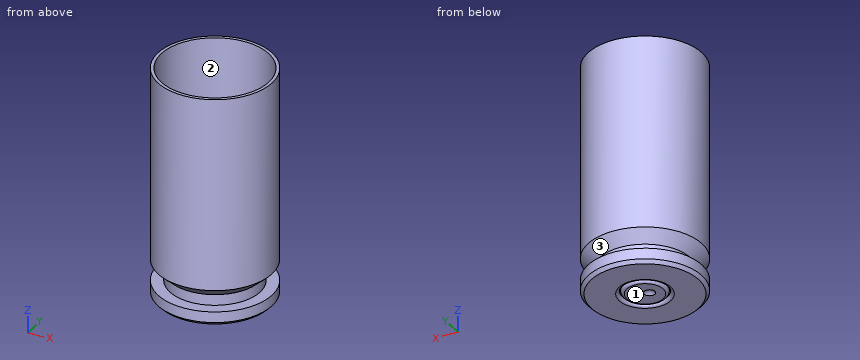
from build123d import *

# Parameters (mm, degrees)
F2_R    = 2
F3_R    = 0.3
F4_SIZE = 0.3


with BuildPart() as f1:
    # F0 (on Front) → F1 (revolve)
    with BuildSketch(Plane.XZ):
        Polygon((2.1, 0), (5.3, 0), (5.3, 1.3), (4.2, 1.3), (4.2, 2.3), (5.3, 3.3), (5.3, 21.25), (5, 21.25), (5, 3.378872), (0.63314, 3.378872), (0.63314, 1.22387), (0, 1.22387), (0, 0), (2, 0), (2, 0.961065), (2.1, 0.961065), align=None)
    revolve(axis=Axis((0, 0, 10.625), (0, 0, 1)))

    # F2
    f2_edges = [f1.edges().sort_by_distance(p)[0] for p in [
        (-5, 0, 3.378872),
    ]]
    fillet(f2_edges, radius=F2_R)

    # F3
    f3_edges = [f1.edges().sort_by_distance(p)[0] for p in [
        (-2.1, 0, 0),
        (-2, 0, 0),
    ]]
    fillet(f3_edges, radius=F3_R)

    # F4
    f4_edges = [f1.edges().sort_by_distance(p)[0] for p in [
        (-5.3, 0, 0),
    ]]
    chamfer(f4_edges, length=F4_SIZE)

    # F5 (on Front) → F6 (revolve, cut)
    with BuildSketch(Plane.XZ):
        with BuildLine():
            Line((-0.916817, 0), (-0.416817, 0))
            Line((-0.416817, 0), (-0.416817, 0.205113))
            ThreePointArc((-0.416817, 0.205113), (-0.687035, 0.151842), (-0.916817, 0))
        make_face()
    revolve(axis=Axis((-0.416817, 0, 0.102557), (0, 0, 1)), mode=Mode.SUBTRACT)


solid = f1.part
Design review of the part built by this model. Coordinates are the model's own, in mm. Face numbers are marked on the shaded views. Coordinates: 2 decimals unless noted, no trailing zeros. Write each loop counter-clockwise with the first axis right and the second up, starting at its lowest first coordinate (ties: lowest second). Pieces come first, ordered by that corner, then holes. Notation, with made-up numbers: (3.5, -21) - (46.5, -21) arc R10 cw to (46.5, -11) - close; hole circle Ø7 at (22.25, -15.5). An arc over 180 degrees is marked (long way). One line per item, written item: value.
1) Add section B-B (z = 4.5). State the section outline as (x, y) points.
Answer sheet:
outline: circle Ø10.6 at (0, 0); hole circle Ø9.59 at (0, 0)
2) Add section A-A (z = 17.25). State the section outline as (x, y) points.
Answer sheet:
outline: circle Ø10.6 at (0, 0); hole circle Ø10 at (0, 0)
3) To check wall thickness, follow probe 1 along Y at (x, z) = (0, 10.25); probe 2 along Z at (x, y) = (-1.25, -2); probe 3 along Y at (x, z) = (3, 19.25). State the ranges of each line that lie inside material, in increasing order.
Answer sheet:
probe 1: y = -5.3 to -5, 5 to 5.3
probe 2: z = 0 to 3.38
probe 3: y = -4.37 to -4, 4 to 4.37
4) Insertion check: pin 1 (3.5 mm diameter, centred on x = 0, y = 0, fed in from +Z); pin 2 (6 mm diameter, centred on x = -1.5, y = 2, fed in from +Z); pin 3 (2 mm diameter, centred on x = 1.5, z = 18, fed in from +Y); pin 4 (5.5 mm diameter, centred on x = 1.5, y = -0.5, fed in from +Z). Each pin has a flat end and moves straight along its axis. Give the tip position at first contact, or say it passes through.
Answer sheet:
pin 1: stops at z = 3.38
pin 2: stops at z = 21.25
pin 3: stops at y = 5.28
pin 4: stops at z = 3.89
5) Mouldability with a two-part tool opening along Z and no side actions: class the marked faces 1, 2 and 3 as +Z half, -Z half, draft (parallel to the pull), parting line (faces both ways), or undercut.
Answer sheet:
face 1: -Z half
face 2: draft
face 3: undercut
